```python
from build123d import *

# Parameters (mm, degrees)
BOSS_EXTRUDE1_DEPTH      = 4.875
BOSS_EXTRUDE1_DEPTH_BACK = 4.875
SKETCH3_R                = 1.1
CUT_EXTRUDE1_DEPTH       = 6.11718917
FILLET1_R                = 0.078539816
CIRPATTERN1_COUNT        = 9
FILLET1_OF_CIRPATTERN1_R = 0.078539816
SKETCH5_W                = 0.95
SKETCH5_H                = 0.86


with BuildPart() as part:
    # Sketch3 → Boss-Extrude1 (new, two sides: drawn at the far end of the back side and taken through both)
    with BuildSketch(Plane.XY.offset(-BOSS_EXTRUDE1_DEPTH_BACK)):
        Circle(SKETCH3_R)
    extrude(amount=BOSS_EXTRUDE1_DEPTH + BOSS_EXTRUDE1_DEPTH_BACK)

    # Sketch4 → Cut-Extrude1 (cut, symmetric)
    with BuildSketch(Plane.XY):
        with BuildLine():
            Line((0.645237551, -0.078539816), (0.645237551, 0.078539816))
            ThreePointArc((0.645237551, 0.078539816), (0.876414028, 0.153933636), (1.051662121, 0.322500826))
            ThreePointArc((1.051662121, 0.322500826), (1.1, 0), (1.051662121, -0.322500826))
            ThreePointArc((1.051662121, -0.322500826), (0.876414028, -0.153933636), (0.645237551, -0.078539816))
        make_face()
    cut_extrude1 = extrude(amount=CUT_EXTRUDE1_DEPTH, both=True, mode=Mode.SUBTRACT)

    # Fillet1
    fillet1_edges = [part.edges().sort_by_distance(p)[0] for p in [
        (0.645237551, 0.078539816, 0),
        (0.645237551, -0.078539816, 0),
    ]]
    fillet(fillet1_edges, radius=FILLET1_R)

    # CirPattern1: Cut-Extrude1 ×9 about axis
    cirpattern1_axis = Axis((0, 0, 0), (0, 0, 1))
    for i in range(1, CIRPATTERN1_COUNT):
        add(cut_extrude1.rotate(cirpattern1_axis, i * 360 / CIRPATTERN1_COUNT), mode=Mode.SUBTRACT)

    # Fillet1 of CirPattern1
    fillet1_of_cirpattern1_edges = [part.edges().sort_by_distance(p)[0] for p in [
        (0.44379622, 0.474915693, 0),
        (0.544765061, 0.354585713, 0),
        (0.034697705, 0.649073239, 0),
        (0.189390945, 0.621796647, 0),
        (-0.390636252, 0.519522202, 0),
        (-0.254601299, 0.598062019, 0),
        (-0.633187165, 0.146880954, 0),
        (-0.579462766, 0.294487526, 0),
        (-0.579462766, -0.294487526, 0),
        (-0.633187165, -0.146880954, 0),
        (-0.254601299, -0.598062019, 0),
        (-0.390636252, -0.519522202, 0),
        (0.189390945, -0.621796647, 0),
        (0.034697705, -0.649073239, 0),
        (0.544765061, -0.354585713, 0),
        (0.44379622, -0.474915693, 0),
    ]]
    fillet(fillet1_of_cirpattern1_edges, radius=FILLET1_OF_CIRPATTERN1_R)

    # Sketch5 → Cut-Revolve1 (revolve, cut)
    with BuildSketch(Plane(origin=(0, 0, 0), x_dir=(0, 0, -1), z_dir=(1, 0, 0)), mode=Mode.PRIVATE) as cut_revolve1_sk:
        Polygon((4.875, 1.3), (4.875, 0.44), (3.925, 0.44), (3.925, 0.6), (1.875, 0.6), (1.875, 0.875), (-0.825, 0.875), (-0.825, 1.3), align=None)
        with Locations((-4.4, 0.87)):
            Rectangle(SKETCH5_W, SKETCH5_H)
    revolve(cut_revolve1_sk.sketch.rotate(Axis((0, 0, 4.875), (0, 0, -1)), 90), axis=Axis((0, 0, 4.875), (0, 0, -1)), mode=Mode.SUBTRACT)


solid = part.part
```
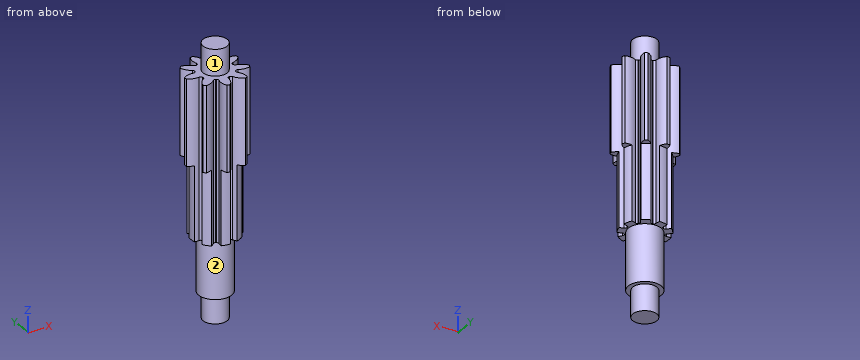
The listing builds one solid part. Answer for the finished solid, in the listing's coordinates (mm). Face numbers are marked on the shaded views. A direction names the side the tool comes from. Round coordinates to 2 decimals unless told otherwise and drop trailing zeros. Loops run counter-clockwise (first coordinate to the right, second up) from the corner with the lowest first, then second, coordinate; pieces in that order, holes last.
Q1. Find the intervals of material crossed by line 1 (Y direction, x = -0.75, z = 1.5); line 2 (Z direction, x = 0.3, y = 0.4) (3 decimals); line 3 (Z direction, x = 0.65, y = -0.1) (3 decimals), in increasing order.
Q2. Which of the six approach directions +Z, -Z, +X, -X, +Y, -Y give full straight-line access (tool end or side, diameter ignored) to the marked faces 1 and 2?
Q3. Section A-A, the plane z = 4.25 is taken. Determine the outline of the cut face in (x, y), then the cut area to 3 significant figures.
Q4. Section B-B, the plane z = -3.75 is taken. Determine the outline of the cut face in (x, y), then the cut area to 3 significant figures.
Completed:
1. line 1: y = -0.74 to -0.42, -0.16 to 0.16, 0.42 to 0.74
1. line 2: z = -3.925 to 3.925
1. line 3: z = -1.875 to 3.925
2. face 1: +Z
2. face 2: -Z
3. outline: circle Ø0.88 at (0, 0)
3. area: 0.608 mm2
4. outline: circle Ø1.2 at (0, 0)
4. area: 1.13 mm2
